The model under review builds one solid part; all positions refer to its coordinate system, in mm. Face numbers are marked on the shaded views. A direction names the side the tool comes from. Give positions to 0.01 mm unless a question says otherwise; leave off trailing zeros. Order: outer loops, then holes, each group sorted by start corner. A loop starts at its lowest first (then second) coordinate and runs counter-clockwise, first axis right, second up.
```python
from build123d import *

# Parameters (mm, degrees)
F1_DEPTH = 63.5
F3_DEPTH = 25.4
F5_DEPTH = 25.4
F7_DEPTH = 50.801


with BuildPart() as f1:
    # F0 (on Top) → F1 (new body)
    with BuildSketch(Plane.XY):
        Polygon((-21.019149, 87.15245), (-97.219149, 87.15245), (-97.219149, 23.65245), (-71.819149, 23.65245), (-71.819149, -27.14755), (-46.419149, -27.14755), (-46.419149, 23.65245), (-21.019149, 23.65245), align=None)
    extrude(amount=F1_DEPTH)

    # F2 (on face) → F3 (cut)
    with BuildSketch(Plane(origin=(-97.219149, 0, 0), x_dir=(0, -1, 0), z_dir=(-1, 0, 0))):
        Polygon((-23.65245, 63.5), (-49.05245, 63.5), (-23.65245, 0), align=None)
    extrude(amount=-F3_DEPTH, mode=Mode.SUBTRACT)

    # F4 (on face) → F5 (cut)
    with BuildSketch(Plane.YZ.offset(-21.019149)):
        Polygon((23.65245, 0), (49.05245, 63.5), (23.65245, 63.5), align=None)
    extrude(amount=-F5_DEPTH, mode=Mode.SUBTRACT)

    # F6 (on face) → F7 (cut, through all)
    with BuildSketch(Plane.YZ.offset(-46.419149)):
        Polygon((-27.14755, 0), (-5.36292, 63.5), (-27.14755, 63.5), align=None)
    extrude(amount=-F7_DEPTH, mode=Mode.SUBTRACT)


solid = f1.part
```
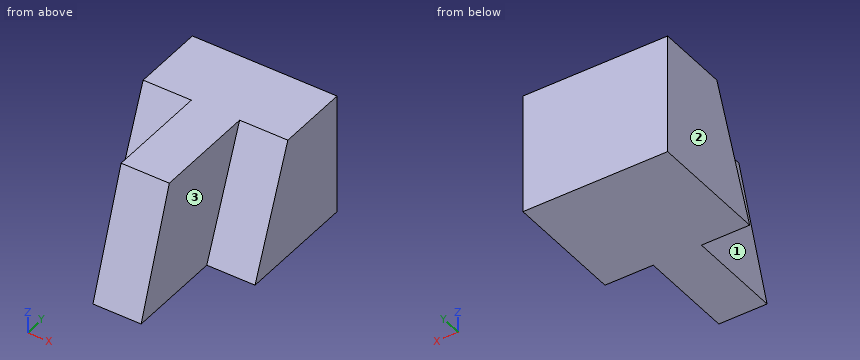
Item 1: For line 1 (X direction, y = 22, z = 16); line 2 (Y direction, x = -65, z = 38); line 3 (Y direction, x = -32, z = 35), list the stretches that pass through material, from the lowest coordinate up.
Values found:
line 1: x = -71.82 to -46.42
line 2: y = -14.11 to 87.15
line 3: y = 37.65 to 87.15
Item 2: For the marked faces 1, 2 and 3, list the 3-axis set-ups (+Z, -Z, +X, -X, +Y, -Y) from which the entire face can be reached by the end or side of a thin tool; tool diameter is ignored.
Values found:
face 1: +Z, -X, -Y
face 2: +Z, -Z, -X, +Y, -Y
face 3: +Z, +X, -Y
Item 3: Take a section at D-D (x = -44.5). Give the boundary of the cut face in (y, z), and give its area (3 significant figures).
Values found:
outline: (23.65, 0) - (87.15, 0) - (87.15, 63.5) - (49.05, 63.5) - close
area: 3,230 mm2
Item 4: Take a section at B-B (y = 38.5). Give the boundary of the cut face in (x, z), and give its area (3 significant figures).
Values found:
outline: (-97.22, 0) - (-21.02, 0) - (-21.02, 37.12) - (-46.42, 37.12) - (-46.42, 63.5) - (-71.82, 63.5) - (-71.82, 37.12) - (-97.22, 37.12) - close
area: 3,500 mm2
Item 5: Clearance check with flat-ended pins moving along their axes: pin 1 Ø1 at (x, z) = (-42, 36) entering from -Y; pin 2 Ø19 at (y, z) = (-4, 39) entering from +X; pin 3 Ø12 at (y, z) = (-9, 46) entering from -X. State where each tip first meets the part, or that it passes through.
Values found:
pin 1: stops at y = 37.85
pin 2: stops at x = -46.42
pin 3: stops at x = -71.82
Item 6: Take a section at A-A (z = 13.5). Give the boundary of the cut face in (x, y), and give its area (3 significant figures).
Values found:
outline: (-97.22, 29.05) - (-71.82, 29.05) - (-71.82, -22.52) - (-46.42, -22.52) - (-46.42, 29.05) - (-21.02, 29.05) - (-21.02, 87.15) - (-97.22, 87.15) - close
area: 5,740 mm2
Item 7: Take a section at C-C (x = -59.5). Give the boundary of the cut face in (y, z).
Values found:
outline: (-27.15, 0) - (87.15, 0) - (87.15, 63.5) - (-5.36, 63.5) - close
